Source: CAD feature listing. Evaluate the final solid. Frame: model axes, mm. Face numbers are marked on the shaded views. A direction names the side the tool comes from. Give positions to 0.01 mm unless a question says otherwise; leave off trailing zeros. Order: outer loops, then holes, each group sorted by start corner. A loop starts at its lowest first (then second) coordinate and runs counter-clockwise, first axis right, second up. Notation, with made-up numbers: M -10,84.5 L 42,84.5 A18 ccw 42,116.5 Z; hole C 14.5,41.5 d7. An arc over 180 degrees is marked long. Answer in a Markdown table with one row per item. Add a question column.
(1) Section query B-B, the plane x = 91. Return loops of the section in (y, z), plus the area to 3 significant figures.
(2) Set-up query: the marked faces 4, 5 and 6. Return all of +Z, -Z, +X, -X, +Y, -Y with unobstructed straight access to the full face (end or side cutting, diameter ignored); none if empty.
(3) Pin query (flat end, axial travel): P1, Ø3, axis at x = 81.5, z = 3, coming from the +Y side; P2, Ø1.9, axis at y = 27, z = 3.5, coming from the +X side; P3, Ø10, axis at x = 92.5, y = 14.5, coming from the -Z side; P4, Ø1.3, axis at y = 12, z = 2.5, coming from the -X side. Return the tip coordinate at first contact, or that it passes through.
(4) Section query A-A, the plane x = 65. Return loops of the section in (y, z), plus the area to 3 significant figures.
(5) Section query D-D, the plane z = 4. Count the separate pieces of the cut face and the enclosed holes in it, plus the area to 3 significant figures.
(6) Material intervals for line 1 along Y through (x, z) = (51, 3); line 2 along Y through (x, z) = (40, 2.5); line 3 along X through (y, z) = (9, 5.75) (3 decimals), sorted ascending.
(7) Mould query, pull axis X, two halves, no side actions, for the marked faces 1, 2 and 3. Classes: pulls with the +X half, pulls with the -X half, needs draft (parallel to the pull), parting line crosses it, or undercut.
(8) Section query C-C, the plane x = 104. Return loops of the section in (y, z) (3 decimals), plus the area to 3 significant figures.
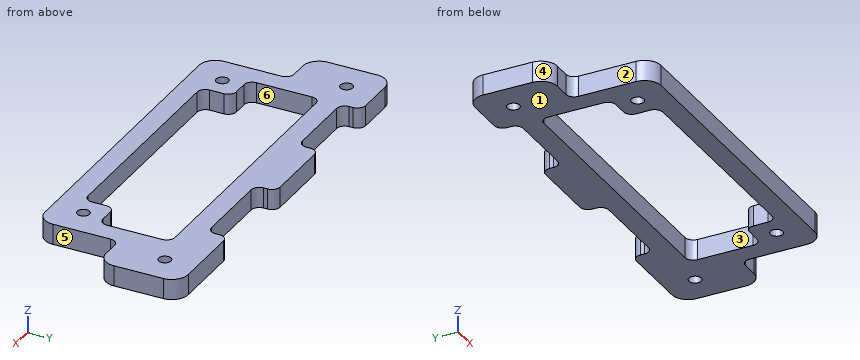
from build123d import *

# Parameters (mm, degrees)
SKETCH1_R           = 1.89865
SKETCH1_R_2         = 1.5875
BOSS_EXTRUDE1_DEPTH = 6.35
FILLET1_R           = 5.08
FILLET2_R           = 2.54
SKETCH2_W           = 25.4
SKETCH2_H           = 6.35
SKETCH2_W_2         = 28.575
CUT_EXTRUDE1_DEPTH  = 8.89
FILLET3_R           = 2.54


with BuildPart() as part:
    # Sketch1 → Boss-Extrude1 (new body)
    with BuildSketch(Plane.XY):
        Polygon((0, 50.8), (0, 25.4), (12.7, 25.4), (12.7, 0), (114.3, 0), (114.3, 25.4), (127, 25.4), (127, 50.8), align=None)
        with Locations((22.225, 9.525)):
            Circle(SKETCH1_R, mode=Mode.SUBTRACT)
        with Locations((52.324, 19.558)):
            Circle(SKETCH1_R_2, mode=Mode.SUBTRACT)
        with Locations((104.775, 9.525)):
            Circle(SKETCH1_R, mode=Mode.SUBTRACT)
        with Locations((52.324, 30.734)):
            Circle(SKETCH1_R_2, mode=Mode.SUBTRACT)
        with Locations((9.525, 41.275)):
            Circle(SKETCH1_R, mode=Mode.SUBTRACT)
        with Locations((23.622, 47.625)):
            Circle(SKETCH1_R_2, mode=Mode.SUBTRACT)
        with Locations((38.1, 47.625)):
            Circle(SKETCH1_R_2, mode=Mode.SUBTRACT)
        with Locations((78.74, 47.625)):
            Circle(SKETCH1_R_2, mode=Mode.SUBTRACT)
        with Locations((89.662, 47.625)):
            Circle(SKETCH1_R_2, mode=Mode.SUBTRACT)
        with Locations((117.475, 41.275)):
            Circle(SKETCH1_R, mode=Mode.SUBTRACT)
    extrude(amount=BOSS_EXTRUDE1_DEPTH)

    # Fillet1
    fillet1_edges = [part.edges().sort_by_distance(p)[0] for p in [
        (114.3, 0, 3.175),
        (12.7, 0, 3.175),
        (0, 25.4, 3.175),
        (0, 50.8, 3.175),
        (127, 50.8, 3.175),
        (127, 25.4, 3.175),
    ]]
    fillet(fillet1_edges, radius=FILLET1_R)

    # Fillet2
    fillet2_edges = [part.edges().sort_by_distance(p)[0] for p in [
        (12.7, 25.4, 3.175),
        (114.3, 25.4, 3.175),
    ]]
    fillet(fillet2_edges, radius=FILLET2_R)

    # Sketch2 → Cut-Extrude1 (cut)
    with BuildSketch(Plane.XY.offset(6.35)):
        with Locations((31.75, 47.625)):
            Rectangle(SKETCH2_W, SKETCH2_H)
        with Locations((84.1375, 47.625)):
            Rectangle(SKETCH2_W_2, SKETCH2_H)
        Polygon((19.05, 38.1), (19.05, 15.875), (28.575, 15.875), (28.575, 6.35), (98.425, 6.35), (98.425, 15.875), (107.95, 15.875), (107.95, 38.1), align=None)
    extrude(amount=-CUT_EXTRUDE1_DEPTH, mode=Mode.SUBTRACT)

    # Fillet3
    fillet3_edges = [part.edges().sort_by_distance(p)[0] for p in [
        (19.05, 50.8, 3.175),
        (44.45, 50.8, 3.175),
        (44.45, 44.45, 3.175),
        (19.05, 44.45, 3.175),
        (69.85, 50.8, 3.175),
        (98.425, 50.8, 3.175),
        (98.425, 44.45, 3.175),
        (69.85, 44.45, 3.175),
        (19.05, 38.1, 3.175),
        (107.95, 38.1, 3.175),
        (107.95, 15.875, 3.175),
        (98.425, 15.875, 3.175),
        (98.425, 6.35, 3.175),
        (28.575, 6.35, 3.175),
        (28.575, 15.875, 3.175),
        (19.05, 15.875, 3.175),
    ]]
    fillet(fillet3_edges, radius=FILLET3_R)


solid = part.part
Values follow:
| question | item | result |
|---|---|---|
| 1 | outline | M 0,0 L 6.35,0 L 6.35,6.35 L 0,6.35 Z; M 38.1,0 L 44.45,0 L 44.45,6.35 L 38.1,6.35 Z |
| 1 | area | 80.6 mm² |
| 2 | face 4 | +Z, -Z, -X, -Y |
| 2 | face 5 | +Z, -Z, +X, -Y |
| 2 | face 6 | +Z, -Z |
| 3 | P1 | stops at y = 44.45 |
| 3 | P2 | stops at x = 126.33 |
| 3 | P3 | passes through |
| 3 | P4 | stops at x = 12.7 |
| 4 | outline | M 0,0 L 6.35,0 L 6.35,6.35 L 0,6.35 Z; M 38.1,0 L 50.8,0 L 50.8,6.35 L 38.1,6.35 Z |
| 4 | area | 121 mm² |
| 5 | separate pieces | 1 |
| 5 | enclosed holes | 5 |
| 5 | area | 2,750 mm² |
| 6 | line 1 | y = 0 to 6.35, 38.1 to 50.8 |
| 6 | line 2 | y = 0 to 6.35, 38.1 to 44.45 |
| 6 | line 3 | x = 12.7 to 20.4, 24.05 to 28.575, 98.425 to 102.95, 106.6 to 114.3 |
| 7 | face 1 | needs draft |
| 7 | face 2 | pulls with the -X half |
| 7 | face 3 | undercut |
| 8 | outline | M 0,0 L 7.792,0 L 7.792,6.35 L 0,6.35 Z; M 11.258,0 L 15.875,0 L 15.875,6.35 L 11.258,6.35 Z; M 38.1,0 L 50.8,0 L 50.8,6.35 L 38.1,6.35 Z |
| 8 | area | 159 mm² |
